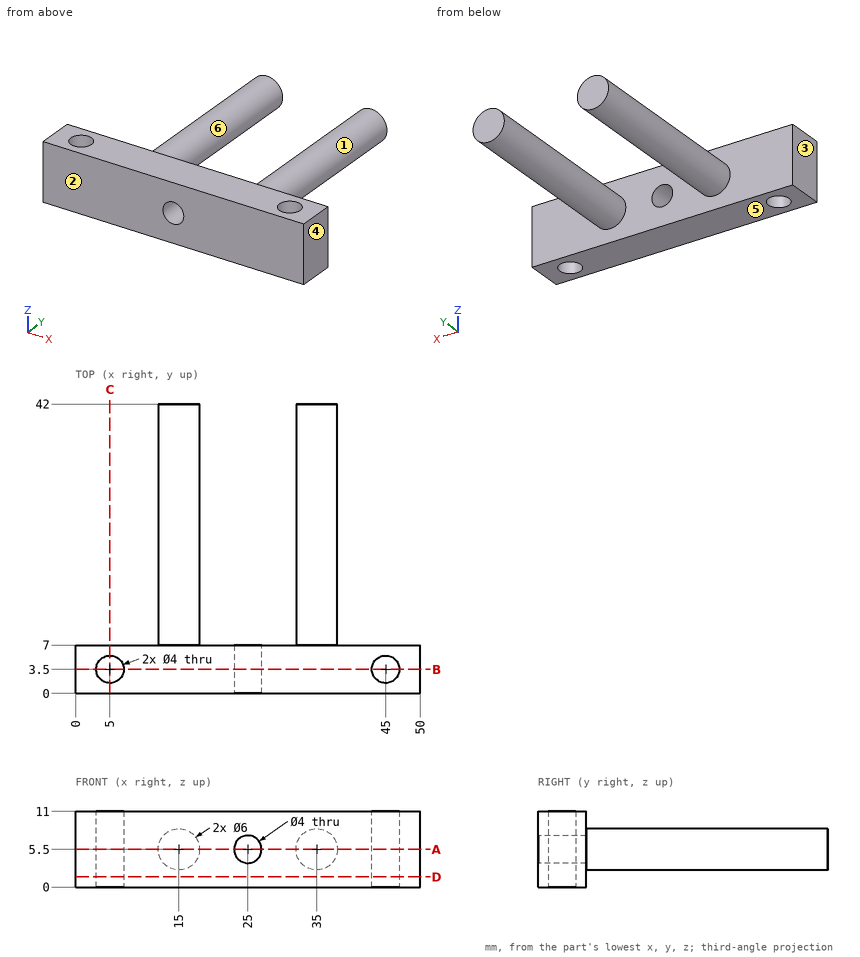
Job drawing, mm, ordinate dimensions from the low corner. One solid piece. A direction names the side the tool comes from. Coordinates: 2 decimals unless noted, no trailing zeros. Write each loop counter-clockwise with the first axis right and the second up, starting at its lowest first coordinate (ties: lowest second). Pieces come first, ordered by that corner, then holes. Notation, with made-up numbers: M 38.5,20.25 L 63.5,20.25 A17 ccw 63.5,49.25 Z; hole C 75,-20.75 d8. An arc over 180 degrees is marked long. Answer as a JSON object with one key per item and string values. Group by question number.
1) Pin check, flat tips, straight feed: pin 1 Ø2 at (x, y) = (35.5, 28.5) entering from +Z; pin 2 Ø5 at (x, y) = (5, 3.5) entering from +Z; pin 3 Ø2 at (x, y) = (15.5, 34) entering from -Z; pin 4 Ø10 at (x, y) = (42, 31) entering from +Z. Stop position of each tip, or through.
2) Wall check: line 1 (X direction, y = 15, z = 5.25); line 2 (Y direction, x = 45, z = 8.75); line 3 (Z direction, x = 25, y = 5.75). Give the ranges that are in metal, low to high. Write a range as from..to.
3) Mould opens along X. For the marked faces 1, 2, 3 and 4 say: +X half, -X half, draft (parallel to the pull), parting line (faces both ways), or undercut.
4) Tool access for the marked faces 5 and 6: list every direction of +Z, -Z, +X, -X, +Y, -Y with a clear straight run to the whole face (end or side of a thin tool).
5) Saw through at C-C (x = 5). Write the cut outline in (y, z), plus the area to 3 significant figures.
6) Saw through at A-A (z = 5.5). Write the cut outline in (x, y).
7) Saw through at D-D (z = 1.5). Write the cut outline in (x, y), plus the area to 3 significant figures.
8) Saw through at B-B (y = 3.5). Write the cut outline in (x, z), plus the area to 3 significant figures.
Values follow:
{
 "1": {"pin 1": "stops at z = 8.5", "pin 2": "stops at z = 11", "pin 3": "stops at z = 2.5", "pin 4": "stops at z = 7.74"},
 "2": {"line 1": "x = 12.01..17.99, 32.01..37.99", "line 2": "y = 0..1.5, 5.5..7", "line 3": "z = 0..3.5, 7.5..11"},
 "3": {"face 1": "undercut", "face 2": "draft", "face 3": "-X half", "face 4": "+X half"},
 "4": {"face 5": "-Z, +X, -X, +Y, -Y", "face 6": "+Y"},
 "5": {"outline": "M 0,0 L 1.5,0 L 1.5,11 L 0,11 Z; M 5.5,0 L 7,0 L 7,11 L 5.5,11 Z", "area": "33.0 mm2"},
 "6": {"outline": "M 0,0 L 23,0 L 23,7 L 18,7 L 18,42 L 12,42 L 12,7 L 0,7 Z; M 27,0 L 50,0 L 50,7 L 38,7 L 38,42 L 32,42 L 32,7 L 27,7 Z; hole C 5,3.5 d4; hole C 45,3.5 d4"},
 "7": {"outline": "M 0,0 L 50,0 L 50,7 L 0,7 Z; hole C 5,3.5 d4; hole C 45,3.5 d4", "area": "325 mm2"},
 "8": {"outline": "M 0,0 L 3,0 L 3,11 L 0,11 Z; M 7,0 L 43,0 L 43,11 L 7,11 Z; M 47,0 L 50,0 L 50,11 L 47,11 Z; hole C 25,5.5 d4", "area": "449 mm2"}
}
